Check sheet for the modelled part. Datum: model origin and axes. Units: mm. Face numbers are marked on the shaded views. A direction names the side the tool comes from. Give positions to 0.01 mm unless a question says otherwise; leave off trailing zeros. Order: outer loops, then holes, each group sorted by start corner. A loop starts at its lowest first (then second) coordinate and runs counter-clockwise, first axis right, second up.
Item 1: Access from +Z, -Z, +X, -X, +Y, -Y to the whole of each face (thin tool, end or side, straight path). Record for the marked faces 4, 5 and 6.
Item 2: Release check for a two-part mould opening along Z. For the marked faces 1, 2 and 3 record: released by +Z, released by -Z, zero draft, split by the parting line, or undercut.
Item 3: Sectioned sample at B-B on x = 0. Record the boundary of the cut face in (y, z).
Item 4: Material ranges on line 1 along X through (y, z) = (-0.3, 0); line 2 along Z through (x, y) = (0, -0.75); line 3 along Z through (x, y) = (0, -0.25), recorded low to high.
Item 5: Sectioned sample at C-C on y = -1.9. Record the boundary of the cut face in (x, z).
Item 6: Gauge pin test, flat ends, axial feed: P1, Ø1, axis at x = 1, y = -1, coming from the +Z side; P2, Ø2.5, axis at x = -23, z = 0, coming from the -Y side; P3, Ø4, axis at x = -23, z = 0, coming from the -Y side; P4, Ø4, axis at x = -13.5, z = 1, coming from the -Y side. Record the tip position at first contact, or that the pin passes through.
Item 7: Sectioned sample at A-A on z = 0. Count the separate pieces of the cut face and the enclosed holes in it, and give its area (3 significant figures).
Item 8: Sectioned sample at D-D on x = -11.25. Record the boundary of the cut face in (y, z), and give its area (3 significant figures).
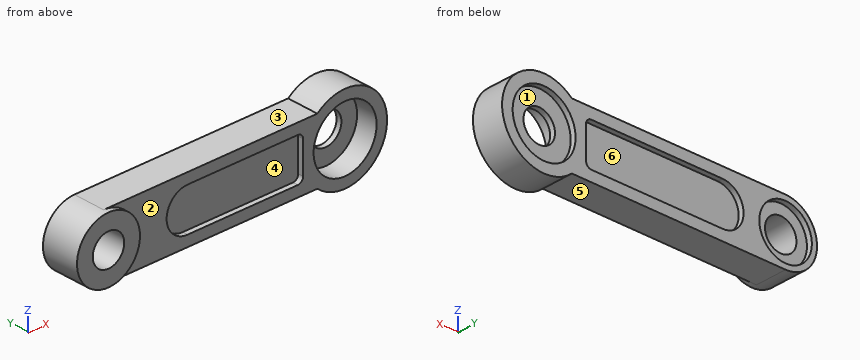
from build123d import *

# Parameters (mm, degrees)
SKETCH1_R           = 4
BOSS_EXTRUDE1_DEPTH = 3
SKETCH5_W           = 23
SKETCH5_H           = 6
BOSS_EXTRUDE2_DEPTH = 3
SKETCH2_R           = 3
CUT_EXTRUDE4_DEPTH  = 0.5
SKETCH7_R           = 1.5
CUT_EXTRUDE5_DEPTH  = 3.5
SKETCH8_R           = 3
CUT_EXTRUDE7_DEPTH  = 2
SKETCH9_R           = 3
BOSS_EXTRUDE3_DEPTH = 3
SKETCH10_R          = 2.5
CUT_EXTRUDE8_DEPTH  = 0.5
CUT_EXTRUDE10_DEPTH = 0.5
CUT_EXTRUDE11_DEPTH = 0.5
SKETCH11_R          = 3
BOSS_EXTRUDE5_DEPTH = 0.5
SKETCH15_R          = 1.5
CUT_EXTRUDE12_DEPTH = 4


with BuildPart() as part:
    # Sketch1 → Boss-Extrude1 (new body)
    with BuildSketch(Plane(origin=(0, 0, 0), x_dir=(1, 0, 0), z_dir=(0, 1, 0))):
        Circle(SKETCH1_R)
    extrude(amount=-BOSS_EXTRUDE1_DEPTH)

    # Sketch5 → Boss-Extrude2 (add)
    with BuildSketch(Plane(origin=(0, 0, 0), x_dir=(1, 0, 0), z_dir=(0, 1, 0))):
        with Locations((-11.5, 0)):
            Rectangle(SKETCH5_W, SKETCH5_H)
    extrude(amount=-BOSS_EXTRUDE2_DEPTH)

    # Sketch2 → Cut-Extrude4 (cut)
    with BuildSketch(Plane(origin=(0, 0, 0), x_dir=(1, 0, 0), z_dir=(0, 1, 0))):
        Circle(SKETCH2_R)
    extrude(amount=-CUT_EXTRUDE4_DEPTH, mode=Mode.SUBTRACT)

    # Sketch7 → Cut-Extrude5 (cut, through all)
    with BuildSketch(Plane(origin=(0, -0.5, 0), x_dir=(1, 0, 0), z_dir=(0, 1, 0))):
        Circle(SKETCH7_R)
    extrude(amount=-CUT_EXTRUDE5_DEPTH, mode=Mode.SUBTRACT)

    # Sketch8 → Cut-Extrude7 (cut)
    with BuildSketch(Plane.XZ.offset(3)):
        Circle(SKETCH8_R)
    extrude(amount=-CUT_EXTRUDE7_DEPTH, mode=Mode.SUBTRACT)

    # Sketch9 → Boss-Extrude3 (add)
    with BuildSketch(Plane(origin=(0, 0, 0), x_dir=(1, 0, 0), z_dir=(0, 1, 0))):
        with Locations((-23, 0)):
            Circle(SKETCH9_R)
    extrude(amount=-BOSS_EXTRUDE3_DEPTH)

    # Sketch10 → Cut-Extrude8 (cut)
    with BuildSketch(Plane(origin=(0, 0, 0), x_dir=(1, 0, 0), z_dir=(0, 1, 0))):
        with Locations((-23, 0)):
            Circle(SKETCH10_R)
    extrude(amount=-CUT_EXTRUDE8_DEPTH, mode=Mode.SUBTRACT)

    # Sketch12 → Cut-Extrude10 (cut)
    with BuildSketch(Plane(origin=(0, 0, 0), x_dir=(1, 0, 0), z_dir=(0, 1, 0))):
        with BuildLine():
            Line((-4.5, -2), (-17, -2))
            ThreePointArc((-17, -2), (-19, 0), (-17, 2))
            Line((-17, 2), (-4.5, 2))
            ThreePointArc((-4.5, 2), (-4.146446609, 1.853553391), (-4, 1.5))
            Line((-4, 1.5), (-4, -1.5))
            ThreePointArc((-4, -1.5), (-4.146446609, -1.853553391), (-4.5, -2))
        make_face()
    extrude(amount=-CUT_EXTRUDE10_DEPTH, mode=Mode.SUBTRACT)

    # Sketch13 → Cut-Extrude11 (cut)
    with BuildSketch(Plane.XZ.offset(3)):
        with BuildLine():
            Line((-4.5, -2), (-15, -2))
            ThreePointArc((-15, -2), (-17, 0), (-15, 2))
            Line((-15, 2), (-4.5, 2))
            ThreePointArc((-4.5, 2), (-4.146446609, 1.853553391), (-4, 1.5))
            Line((-4, 1.5), (-4, -1.5))
            ThreePointArc((-4, -1.5), (-4.146446609, -1.853553391), (-4.5, -2))
        make_face()
    extrude(amount=-CUT_EXTRUDE11_DEPTH, mode=Mode.SUBTRACT)

    # Sketch11 → Boss-Extrude5 (add)
    with BuildSketch(Plane(origin=(0, -3, 0), x_dir=(1, 0, 0), z_dir=(0, 1, 0))):
        with Locations((-23, 0)):
            Circle(SKETCH11_R)
    extrude(amount=-BOSS_EXTRUDE5_DEPTH)

    # Sketch15 → Cut-Extrude12 (cut, through all)
    with BuildSketch(Plane(origin=(0, -0.5, 0), x_dir=(1, 0, 0), z_dir=(0, 1, 0))):
        with Locations((-23, 0)):
            Circle(SKETCH15_R)
    extrude(amount=-CUT_EXTRUDE12_DEPTH, mode=Mode.SUBTRACT)


solid = part.part
Report:
1. face 4: -Y
1. face 5: -Z, -X, +Y, -Y
1. face 6: +Y
2. face 1: undercut
2. face 2: zero draft
2. face 3: released by +Z
3. outline: (-3, -4) - (0, -4) - (0, -3) - (-0.5, -3) - (-0.5, -1.5) - (-1, -1.5) - (-1, -3) - (-3, -3) - close; (-3, 3) - (-1, 3) - (-1, 1.5) - (-0.5, 1.5) - (-0.5, 3) - (0, 3) - (0, 4) - (-3, 4) - close
4. line 1: x = -26 to -25.5, -20.5 to -19, -4 to -3, 3 to 4
4. line 2: z = -4 to -1.5, 1.5 to 4
4. line 3: z = -4 to -3, 3 to 4
5. outline: (-23, -3) - (-2.65, -3) arc R4 ccw (long way) to (-2.65, 3) - (-23, 3) arc R3 ccw to start; hole circle Ø3 at (-23, 0); hole circle Ø6 at (0, 0)
6. P1: stops at z = 3.97
6. P2: passes through
6. P3: stops at y = -3.5
6. P4: stops at y = -3
7. separate pieces: 3
7. enclosed holes: 0
7. area: 51.0 mm2
8. outline: (-3, -3) - (0, -3) - (0, -2) - (-0.5, -2) - (-0.5, 2) - (0, 2) - (0, 3) - (-3, 3) - (-3, 2) - (-2.5, 2) - (-2.5, -2) - (-3, -2) - close
8. area: 14.0 mm2
